Could you check a few things on this model? Use its own coordinates, in mm. A direction names the side the tool comes from. Coordinates: 2 decimals unless noted, no trailing zeros. Order: outer loops, then holes, each group sorted by start corner. A loop starts at its lowest first (then second) coordinate and runs counter-clockwise, first axis right, second up. Notation, with made-up numbers: M 7,23.5 L 11,23.5 A19 cw 11,38.5 Z; hole C 3,-34 d7. An arc over 180 degrees is marked long. Write item = value, one per line. Start each with the question number.
Autodesk Fusion 360 part; units mm, degrees
sketch "Skizze1" plane through (0, 0, 0) normal (0, 0, 1) x (1, 0, 0)
  circle A0 centre (0, 0) radius 45
  circle A1 centre (0, 0) radius 57
  line L0 (-93.8803, 0) -> (101.1197, 0) construction
  line L1 (0, 80) -> (0, -75) construction
  circle A2 centre (50.5, 0) radius 1.45
  circle A3 centre (0, 50.5) radius 1.45
  line L2 (-57, 57) -> (57, 57) construction
  line L3 (57, 57) -> (57, -57) construction
  line L4 (57, -57) -> (-57, -57) construction
  line L5 (-57, -57) -> (-57, 57) construction
  circle A4 centre (50.5, 0) radius 2.45
  circle A5 centre (0, 50.5) radius 2.45
  circle A6 centre (-50.5, 0) radius 2.45
  circle A7 centre (-50.5, 0) radius 1.45
  circle A8 centre (0, -50.5) radius 2.45
  circle A9 centre (0, -50.5) radius 1.45
  dimension "d1" = 90
  dimension "d2" = 114
  dimension "d3" = 2.9
  dimension "d4" = 2.9
  dimension "d5" = 6.5
  dimension "d6" = 6.5
  dimension "d7" = 4.9
  dimension "d8" = 4.9
extrude "Extrusion1" add sketch "Skizze1" along normal blind 28 contours A1
extrude "Extrusion2" add sketch "Skizze1" along normal blind 24.5 contours A4 | A5 | A6 | A8
equation "d4 = d3"
equation "d6 = d5"
equation "d8 = d7"
(1) Imagine slicing it at D-D on z = 16. List the corners of the cut face in (x, y) for me, plus the area to 3 significant figures.
(2) Please list where these lines run through material, in increasing order: probe 1 along Y at (x, z) = (0, 27.15); probe 2 along Y at (x, z) = (0, 8); probe 3 along Y at (x, z) = (-20, 25.75). Write a range as from..to.
(3) Imagine slicing it at A-A on x = 0. List the corners of the cut face in (y, z) for me.
(4) Imagine slicing it at B-B on y = -36.5. List the corners of the cut face in (x, z) for me.
(5) For faces 1 (the cylindrical face through (-51.95, -0.06, 12.08)), 2 (the flat face through (1, 49, 24.5)), which set-ups out of +Z, -Z, +X, -X, +Y, -Y let a thin tool reach every point of the face, with its end or its side?
(6) Will these pins go through, and if not, where does the flat tip stop? P1, Ø6, axis at x = 37.5, z = 6.5, coming from the +Y side; P2, Ø5, axis at y = 38, z = 3.5, coming from the -X side; P3, Ø8, axis at x = -4.5, z = 8, coming from the +Y side; P4, Ø2.5, axis at x = 0, y = -50.5, coming from the -Z side.
(7) Imagine slicing it at C-C on x = 50.5. List the corners of the cut face in (y, z) for me, plus the area to 3 significant figures.
(8) Thinking about a two-plate mould opening in Y: for faces 3 (the flat face through (25, -38, 28)), 4 (the cylindrical face through (52.654, 21.831, 13.804)), 5 (the flat face through (-49, -1, 24.5)), which applies, released by +Y, released by -Y, zero draft, split by the parting line, or undercut?
Response:
q1.outline = C 0,0 d114; hole C -50.5,0 d2.9; hole C 0,0 d90; hole C 0,-50.5 d2.9; hole C 0,50.5 d2.9; hole C 50.5,0 d2.9
q1.area = 3,820 mm2
q2.probe_1 = -57..-52.95, -48.05..-45, 45..48.05, 52.95..57
q2.probe_2 = -57..-51.95, -49.05..-45, 45..49.05, 51.95..57
q2.probe_3 = -53.38..-40.31, 40.31..53.38
q3.outline = M -57,0 L -51.95,0 L -51.95,24.5 L -52.95,24.5 L -52.95,28 L -57,28 Z; M -49.05,0 L -45,0 L -45,28 L -48.05,28 L -48.05,24.5 L -49.05,24.5 Z; M 45,0 L 49.05,0 L 49.05,24.5 L 48.05,24.5 L 48.05,28 L 45,28 Z; M 51.95,0 L 57,0 L 57,28 L 52.95,28 L 52.95,24.5 L 51.95,24.5 Z
q4.outline = M -43.78,0 L -26.32,0 L -26.32,28 L -43.78,28 Z; M 26.32,0 L 43.78,0 L 43.78,28 L 26.32,28 Z
q5.face_1 = +Z, -Z
q5.face_2 = +Z
q6.P1 = 45.37
q6.P2 = -44.6
q6.P3 = 57
q6.P4 = through
q7.outline = M -26.43,0 L -1.45,0 L -1.45,24.5 L -2.45,24.5 L -2.45,28 L -26.43,28 Z; M 1.45,0 L 26.43,0 L 26.43,28 L 2.45,28 L 2.45,24.5 L 1.45,24.5 Z
q7.area = 1,390 mm2
q8.face_3 = zero draft
q8.face_4 = split by the parting line
q8.face_5 = undercut
